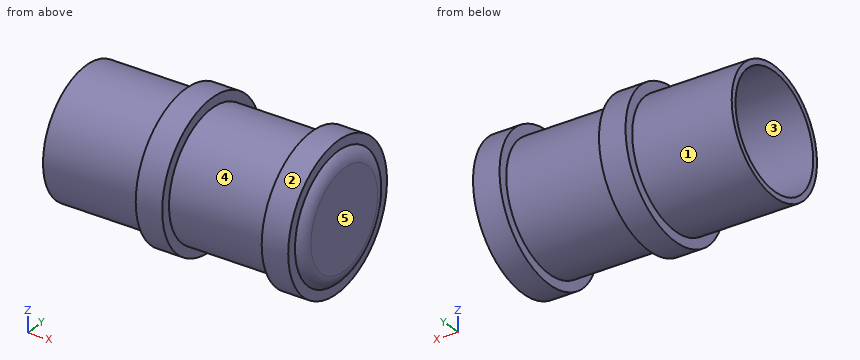
```python
from build123d import *

# Parameters (mm, degrees)
F0_R      = 9.5
F1_DEPTH  = 15
F2_R      = 11
F3_DEPTH  = 4
F4_R      = 9.5
F5_DEPTH  = 15
F6_R      = 11
F7_DEPTH  = 4
F8_R      = 9.5
F9_DEPTH  = 1
F11_R     = 8.65
F12_DEPTH = 36.3
F15_DEPTH = 0.5
F16_DEPTH = 0.5


# Not quite as in the source:
# - a fillet or chamfer that OpenCascade refuses, or shapes differently, is made with other operations: its cross-section is extruded or revolved along the edge and cut away or added


with BuildPart() as f1:
    # F0 (on Right) → F1 (new body)
    with BuildSketch(Plane.YZ):
        Circle(F0_R)
    extrude(amount=F1_DEPTH)

    # F2 (on face) → F3 (join)
    with BuildSketch(Plane.YZ.offset(15)):
        Circle(F2_R)
    extrude(amount=F3_DEPTH)

    # F4 (on face) → F5 (join)
    with BuildSketch(Plane.YZ.offset(19)):
        Circle(F4_R)
    extrude(amount=F5_DEPTH)

    # F6 (on face) → F7 (join)
    with BuildSketch(Plane.YZ.offset(34)):
        Circle(F6_R)
    extrude(amount=F7_DEPTH)

    # F8 (on face) → F9 (join)
    with BuildSketch(Plane.YZ.offset(38)):
        Circle(F8_R)
    extrude(amount=F9_DEPTH)

    # F10: fillet of radius 2.6556349186 on 1 edges, made by hand

    # F10_s1 → F10_t2 (revolve, cut)
    with BuildSketch(Plane.XY):
        with BuildLine():
            ThreePointArc((38, 9.5), (38.7369744021, 8.5759498633), (39, 7.4236402438))
            Line((39, 7.4236402438), (39, 9.5))
            Line((39, 9.5), (38, 9.5))
        make_face()
    revolve(axis=Axis((39, 0, 0), (1, 0, 0)), mode=Mode.SUBTRACT)

    # F11 (on face) → F12 (cut)
    with BuildSketch(Plane(origin=(0, 0, 0), x_dir=(0, -1, 0), z_dir=(-1, 0, 0))):
        Circle(F11_R)
    extrude(amount=-F12_DEPTH, mode=Mode.SUBTRACT)

    # F14 (on Front) → F15 (join, symmetric)
    with BuildSketch(Plane.XZ):
        Polygon((25.5720777049, -8.6574743293), (25.5720777049, 8.6425256707), (24.0004413285, 7.0708892943), (22.4288049522, 8.6425256707), (22.4288049522, -8.6574743293), (24.0004413285, -7.085837953), align=None)
    extrude(amount=F15_DEPTH, both=True)

    # F13 (on Top) → F16 (join, symmetric)
    with BuildSketch(Plane.XY):
        Polygon((24.1439803634, 5.9105833968), (22.2261317603, 8.5902402711), (22.2261317603, -8.7097597289), (24.1439803634, -6.0301028546), (26.0618289666, -8.7097597289), (26.0618289666, 8.5902402711), align=None)
    extrude(amount=F16_DEPTH, both=True)


solid = f1.part
```
Could you check a few things on this model? Use its own coordinates, in mm. Face numbers are marked on the shaded views. A direction names the side the tool comes from. Round coordinates to 2 decimals unless told otherwise and drop trailing zeros. Loops run counter-clockwise (first coordinate to the right, second up) from the corner with the lowest first, then second, coordinate; pieces in that order, holes last. Notation, with made-up numbers: M 26,-18.75 L 66,-18.75 A5 ccw 66,-13.75 Z; hole C -30,85.5 d4. An arc over 180 degrees is marked long. Write item = value, one per line.
1. Which directions (+Z, -Z, +X, -X, +Y, -Y) give clear straight access to the entire face, cutting with the end or side of a thin tool? Please do the marked faces 1 and 2.
Results below:
face_1 = -X
face_2 = +X, -X
2. Thinking about a two-plate mould opening in Z: for the marked faces 3, 4 and 5, which applies, +Z half, -Z half, draft (parallel to the pull), parting line (faces both ways), or undercut?
Results below:
face_3 = undercut
face_4 = parting line
face_5 = draft
3. I want a section at C-C, the plane y = -8. Count the separate pieces of the cut face and the enclosed holes in it, and give its area (3 significant figures).
Results below:
separate_pieces = 3
enclosed_holes = 0
area = 198 mm²
4. I want a section at B-B, the plane x = 29.5. Write out the boundary of the cut face in (y, z), and give its area (3 significant figures).
Results below:
outline = C 0,0 d19; hole C 0,0 d17.3
area = 48.5 mm²
5. Will these pins go through, and if not, where does the flat tip stop? P1, Ø8, axis at x = 7.5, z = -1.5, coming from the +Y side; P2, Ø1.5, axis at x = 21, z = 3, coming from the -Y side; P3, Ø1.2, axis at x = 23, y = 1.5, coming from the -Z side.
Results below:
P1 = 9.5
P2 = -9.23
P3 = -9.46
6. I need wall thicknesses on probe 1 along Z at (x, y) = (26, 0); probe 2 along Z at (x, y) = (18.5, 0); probe 3 along Z at (x, y) = (24.5, -6.25). Which ranges of each line are inside material? Lowest first, please.
Results below:
probe_1 = -9.5 to -8.65, -0.5 to 0.5, 8.65 to 9.5
probe_2 = -11 to -8.65, 8.65 to 11
probe_3 = -7.15 to -5.98, -0.5 to 0.5, 5.98 to 7.15
